from build123d import *

# Parameters (mm, degrees)
SKETCH1_R           = 1.5
BOSS_EXTRUDE1_DEPTH = 10
SKETCH2_R           = 2.25
BOSS_EXTRUDE2_DEPTH = 3
CUT_EXTRUDE1_DEPTH  = 2
CHAMFER1_SIZE       = 0.25
FILLET1_R           = 0.5


with BuildPart() as part:
    # Sketch1 → Boss-Extrude1 (new body)
    with BuildSketch(Plane(origin=(0, 0, 0), x_dir=(1, 0, 0), z_dir=(0, 1, 0))):
        with Locations(Location((0, 0, 0), (0, 0, 270))):
            Circle(SKETCH1_R)
    extrude(amount=BOSS_EXTRUDE1_DEPTH)

    # Sketch2 → Boss-Extrude2 (add)
    with BuildSketch(Plane(origin=(0, 10, 0), x_dir=(1, 0, 0), z_dir=(0, 1, 0))):
        with Locations(Location((0, 0, 0), (0, 0, 270))):
            Circle(SKETCH2_R)
    extrude(amount=BOSS_EXTRUDE2_DEPTH)

    # Sketch3 → Cut-Extrude1 (cut)
    with BuildSketch(Plane(origin=(0, 13, 0), x_dir=(1, 0, 0), z_dir=(0, 1, 0))):
        Polygon((0, 1.154700538), (-1, 0.577350269), (-1, -0.577350269), (0, -1.154700538), (1, -0.577350269), (1, 0.577350269), align=None)
    extrude(amount=-CUT_EXTRUDE1_DEPTH, mode=Mode.SUBTRACT)

    # Chamfer1
    chamfer1_edges = [part.edges().sort_by_distance(p)[0] for p in [
        (0.5, 13, -0.866025404),
        (-0.5, 13, -0.866025404),
        (-1, 13, 0),
        (-0.5, 13, 0.866025404),
        (0.5, 13, 0.866025404),
        (1, 13, 0),
        (0, 10, -2.25),
        (0, 13, -2.25),
    ]]
    chamfer(chamfer1_edges, length=CHAMFER1_SIZE)

    # Fillet1
    fillet1_edges = [part.edges().sort_by_distance(p)[0] for p in [
        (0, 0, -1.5),
    ]]
    fillet(fillet1_edges, radius=FILLET1_R)


solid = part.part
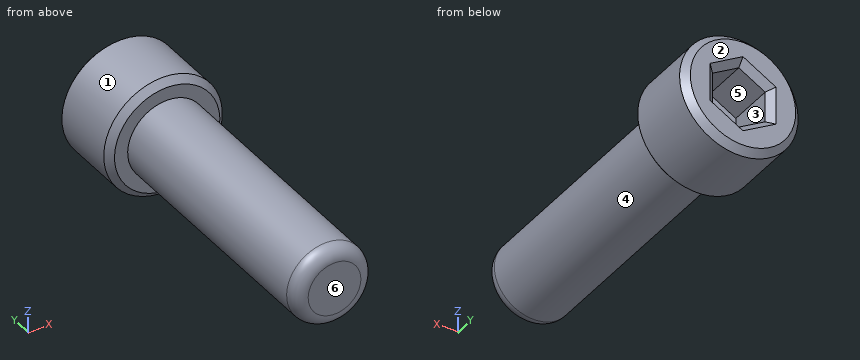
Here's how the part is built. I have some questions about the finished solid (model axes, mm). Face numbers are marked on the shaded views. A direction names the side the tool comes from. Round coordinates to 2 decimals unless told otherwise and drop trailing zeros. Loops run counter-clockwise (first coordinate to the right, second up) from the corner with the lowest first, then second, coordinate; pieces in that order, holes last. Notation, with made-up numbers: (50.25, -40) - (101.25, -40) arc R28 cw to (101.25, -8) - close; hole circle Ø4 at (-39, -7). An arc over 180 degrees is marked (long way). One line per question, with ' | ' between items. Start each with the question number.
Q1. I want a section at C-C (y = 9.5). Write out the boundary of the cut face in (x, z), then the cut area to 3 significant figures.
Q2. Please list where these lines run through material, in increasing order: line 1 (Y direction, x = -1.3, z = 1.05); line 2 (Z direction, x = 0.3, y = 11.25); line 3 (Y direction, x = -0.8, z = -0.3). Write a range as [from, to].
Q3. We'd pull the mould along Z, two halves only. Please class the marked faces 1, 2 and 3: +Z half, -Z half, draft (parallel to the pull), parting line (faces both ways), or undercut.
Q4. I want a section at A-A (y = 11.5). Write out the boundary of the cut face in (x, z), then the cut area to 3 significant figures.
Q5. I want a section at B-B (z = 0). Write out the boundary of the cut face in (x, y).
Q6. For the marked faces 4, 5 and 6, which set-ups out of +Z, -Z, +X, -X, +Y, -Y let a thin tool reach every point of the face, with its end or its side?
Q7. Will these pins go through, and if not, where does the flat tip stop? pin 1 (1.5 mm diameter, centred on x = 0.5, y = 8, fed in from -Z); pin 2 (2 mm diameter, centred on x = 0.5, z = -1, fed in from +Y); pin 3 (1 mm diameter, centred on x = 0, z = 0, fed in from +Y); pin 4 (2 mm diameter, centred on x = -1.5, y = 4, fed in from +Z).
Response values:
1) outline: circle Ø3 at (0, 0) | area: 7.07 mm²
2) line 1: y = [10, 13] | line 2: z = [-2.23, -0.98], [0.98, 2.23] | line 3: y = [0, 11]
3) face 1: parting line | face 2: draft | face 3: undercut
4) outline: circle Ø4.5 at (0, 0); hole (-1, -0.58) - (0, -1.15) - (1, -0.58) - (1, 0.58) - (0, 1.15) - (-1, 0.58) - close | area: 12.4 mm²
5) outline: (-2.25, 10.25) - (-2, 10) - (-1.5, 10) - (-1.5, 0.5) arc R0.5 ccw to (-1, 0) - (1, 0) arc R0.5 ccw to (1.5, 0.5) - (1.5, 10) - (2, 10) - (2.25, 10.25) - (2.25, 12.75) - (2, 13) - (1.25, 13) - (1, 12.75) - (1, 11) - (-1, 11) - (-1, 12.75) - (-1.25, 13) - (-2, 13) - (-2.25, 12.75) - close
6) face 4: -Y | face 5: +Y | face 6: +Z, -Z, +X, -X, -Y
7) pin 1: stops at z = -1.5 | pin 2: stops at y = 13 | pin 3: stops at y = 11 | pin 4: stops at z = 1.41
